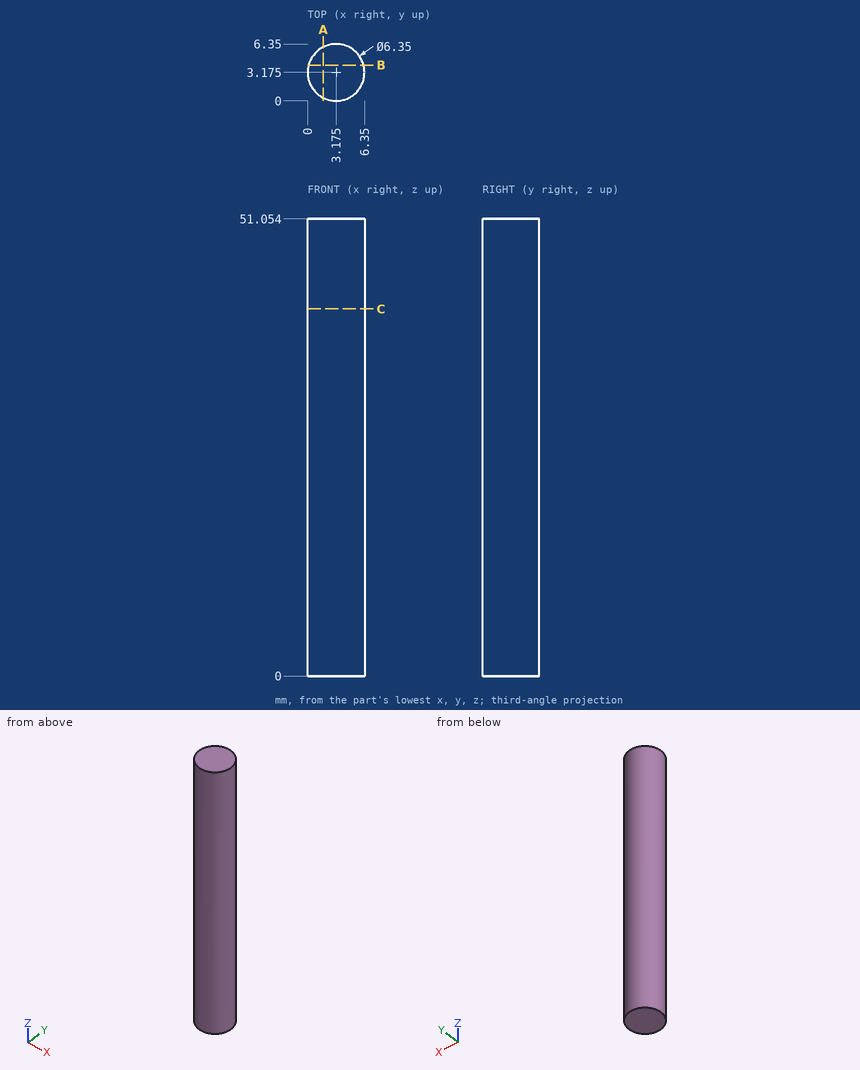
Here's the drawing with two shaded views (mm, measured from the low corner). I have some questions. Give positions to 0.01 mm unless a question says otherwise; leave off trailing zeros. Order: outer loops, then holes, each group sorted by start corner. A loop starts at its lowest first (then second) coordinate and runs counter-clockwise, first axis right, second up. Notation, with made-up numbers: M 38.5,49 L 45.5,49 A25 cw 45.5,62 Z; hole C 21,-20 d5. An arc over 180 degrees is marked long. Answer as a JSON object with one key per item and string values. Group by question number.
1) Suppose I cut it at A-A, the plane x = 1.75. Write out the boundary of the cut face in (y, z).
2) I'm going to push flat-ended pins straight in: pin 1 Ø1 at (x, z) = (5, 29) entering from -Y; pin 2 Ø1 at (y, z) = (3, 31) entering from -X; pin 3 Ø3 at (y, z) = (1, 11.5) entering from -X. Where does each tip first touch, or does it pass through?
3) Suppose I cut it at B-B, the plane y = 4. Write out the boundary of the cut face in (x, z).
4) Please list where these lines run through material, in increasing order: L1, parallel to X at y = 3, z = 26.5; L2, parallel to Y at x = 0.75, z = 4; L3, parallel to X at y = 5.5, z = 7.5. Write a range as [from, to].
5) Suppose I cut it at C-C, the plane z = 41. Write out the boundary of the cut face in (x, y) (3 decimals), plus the area to 3 significant figures.
Results found:
{
 "1": {"outline": "M 0.34,0 L 6.01,0 L 6.01,51.05 L 0.34,51.05 Z"},
 "2": {"pin 1": "y = 0.29", "pin 2": "x = 0", "pin 3": "x = 0.07"},
 "3": {"outline": "M 0.11,0 L 6.24,0 L 6.24,51.05 L 0.11,51.05 Z"},
 "4": {"L1": "[0, 6.35]", "L2": "[1.13, 5.22]", "L3": "[1.01, 5.34]"},
 "5": {"outline": "C 3.175,3.175 d6.35", "area": "31.7 mm²"}
}
